```python
from build123d import *

# Parameters (mm, degrees)
ESQUISSE2_W        = 27.56942971
ESQUISSE2_H        = 25
BOSS_EXTRU_3_DEPTH = 3


with BuildPart() as part:
    # Esquisse2 → Boss.-Extru.3 (new body)
    with BuildSketch(Plane(origin=(0, 0, 0), x_dir=(0, 0, -1), z_dir=(1, 0, 0))):
        with Locations((-243.784714855, 0)):
            Rectangle(ESQUISSE2_W, ESQUISSE2_H)
        Polygon((230, 25), (-230, 25), (-230, 12.5), (-230, -12.5), (-230, -25), (230, -25), (230, -12.6), (207.351490585, -12.6), (207.351490585, 12.6), (230, 12.6), align=None)
    extrude(amount=BOSS_EXTRU_3_DEPTH)


solid = part.part
```
The model under review builds one solid part; all positions refer to its coordinate system, in mm. Give positions to 0.01 mm unless a question says otherwise; leave off trailing zeros. Write each loop counter-clockwise with the first axis right and the second up, starting at its lowest first coordinate (ties: lowest second). Pieces come first, ordered by that corner, then holes.
(1) Consider section B-B, the plane y = -2. Give the boundary of the cut face in (x, z), and give its area (3 significant figures).
(2) To check wall thickness, follow L1, parallel to Z at x = 2, y = -9; L2, parallel to Z at x = 1.8, y = -22. State the ranges of each line that lie inside material, in increasing order.
(3) For P1, Ø0.9, axis at x = 1.5, y = -16, coming from the +Z side, flat-tipped, find the tip position at first contact; note if it passes through.
(4) Consider section A-A, the plane x = 2.05. Give the boundary of the cut face in (y, z), and give its area (3 significant figures).
Returned:
1. outline: (0, -207.35) - (3, -207.35) - (3, 257.57) - (0, 257.57) - close
1. area: 1,390 mm2
2. L1: z = -207.35 to 257.57
2. L2: z = -230 to 230
3. P1: stops at z = 230
4. outline: (-25, -230) - (-12.6, -230) - (-12.6, -207.35) - (12.6, -207.35) - (12.6, -230) - (25, -230) - (25, 230) - (12.5, 230) - (12.5, 257.57) - (-12.5, 257.57) - (-12.5, 230) - (-25, 230) - close
4. area: 23,100 mm2
